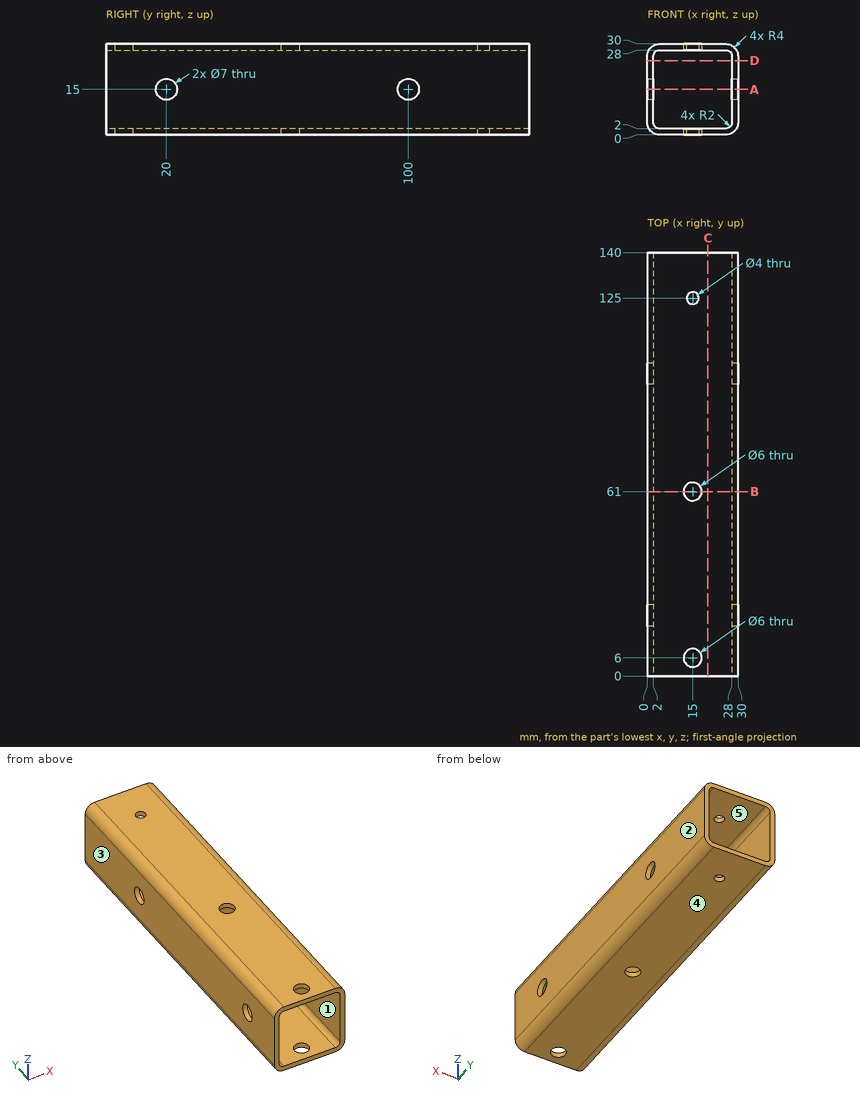
Study the drawing (mm; zero at the part's minimum x, y, z) and answer. A direction names the side the tool comes from. Round coordinates to 2 decimals unless told otherwise and drop trailing zeros. Write each loop counter-clockwise with the first axis right and the second up, starting at its lowest first coordinate (ties: lowest second). Pieces come first, ordered by that corner, then holes. Notation, with made-up numbers: (-27, 81) -> (-12, 81) arc R4 cw to (-12, 88) -> close; hole circle Ø10 at (75.25, -23.5). An arc over 180 degrees is marked (long way). Use CSV: the item, a comma, the result in double quotes. Start each with the question number.
(1) Section C-C on x = 20 is taken. Give the vertices of the cut face in (y, z).
(2) Section B-B on y = 61 is taken. Give the vertices of the cut face in (x, z), then the cut area to 3 significant figures.
(3) Consider L1, parallel to Y at x = 15, z = 1.65; L2, parallel to Z at x = 26, y = 28.5. Determine where each line is inside the solid, lowest interval first. Write a range as from..to.
(4) Section A-A on z = 15 is taken. Give the vertices of the cut face in (x, y), then the cut area to 3 significant figures.
(5) Each of these flat-tipped pins is pushed along its axis until it touches: pin 1 (3 mm diameter, centred on x = 15, y = 125, fed in from +Z); pin 2 (1 mm diameter, centred on x = 12.5, y = 97.5, fed in from -Z). Where does it stop, or does it pass through?
(6) The mould has two halves that part along Z. Classify the marked faces 3, 4 and 5: released by +Z, released by -Z, zero draft, split by the parting line, or undercut.
(7) Which of the six approach directions +Z, -Z, +X, -X, +Y, -Y give full straight-line access (tool end or side, diameter ignored) to the marked faces 1 and 2?
(8) Section D-D on z = 24.5 is taken. Give the vertices of the cut face in (x, y), then the cut area to 3 significant figures.
A:
1,outline,"(0, 0) -> (140, 0) -> (140, 2) -> (0, 2) -> close; (0, 28) -> (140, 28) -> (140, 30) -> (0, 30) -> close"
2,outline,"(0, 4) arc R4 ccw to (4, 0) -> (12, 0) -> (12, 2) -> (4, 2) arc R2 cw to (2, 4) -> (2, 26) arc R2 cw to (4, 28) -> (12, 28) -> (12, 30) -> (4, 30) arc R4 ccw to (0, 26) -> close; (18, 0) -> (26, 0) arc R4 ccw to (30, 4) -> (30, 26) arc R4 ccw to (26, 30) -> (18, 30) -> (18, 28) -> (26, 28) arc R2 cw to (28, 26) -> (28, 4) arc R2 cw to (26, 2) -> (18, 2) -> close"
2,area,"190 mm²"
3,L1,"y = 0..3, 9..58, 64..123, 127..140"
3,L2,"z = 0..2, 28..30"
4,outline,"(0, 0) -> (2, 0) -> (2, 16.5) -> (0, 16.5) -> close; (0, 23.5) -> (2, 23.5) -> (2, 96.5) -> (0, 96.5) -> close; (0, 103.5) -> (2, 103.5) -> (2, 140) -> (0, 140) -> close; (28, 0) -> (30, 0) -> (30, 16.5) -> (28, 16.5) -> close; (28, 23.5) -> (30, 23.5) -> (30, 96.5) -> (28, 96.5) -> close; (28, 103.5) -> (30, 103.5) -> (30, 140) -> (28, 140) -> close"
4,area,"504 mm²"
5,pin 1,"passes through"
5,pin 2,"stops at z = 0"
6,face 3,"zero draft"
6,face 4,"released by -Z"
6,face 5,"undercut"
7,face 1,"+Y, -Y"
7,face 2,"+Z, -Z, +X, +Y, -Y"
8,outline,"(0, 0) -> (2, 0) -> (2, 140) -> (0, 140) -> close; (28, 0) -> (30, 0) -> (30, 140) -> (28, 140) -> close"
8,area,"560 mm²"
